CAD build for the part. Positions are in the model's coordinates, mm. A direction names the side the tool comes from. Give positions to 0.01 mm unless a question says otherwise; leave off trailing zeros. Order: outer loops, then holes, each group sorted by start corner. A loop starts at its lowest first (then second) coordinate and runs counter-clockwise, first axis right, second up.
from build123d import *

# Parameters (mm, degrees)
F0_R     = 4.7625
F0_R_2   = 6.35
F1_DEPTH = 12.7


with BuildPart() as f1:
    # F0 (on Front) → F1 (new body)
    with BuildSketch(Plane.XZ):
        with BuildLine():
            ThreePointArc((8.594672, 44.651487), (8.337428, 45.27728), (8.254523, 45.948784))
            ThreePointArc((8.254523, 45.948784), (0, 54.2925), (-8.254523, 45.948784))
            ThreePointArc((-8.254523, 45.948784), (-8.337428, 45.27728), (-8.594672, 44.651487))
            Line((-8.594672, 44.651487), (-42.966658, -14.882539))
            ThreePointArc((-42.966658, -14.882539), (-43.379988, -15.418216), (-43.920076, -15.825765))
            ThreePointArc((-43.920076, -15.825765), (-47.018684, -27.14625), (-35.665553, -30.123019))
            ThreePointArc((-35.665553, -30.123019), (-35.042561, -29.859064), (-34.371986, -29.768948))
            Line((-34.371986, -29.768948), (34.371986, -29.768948))
            ThreePointArc((34.371986, -29.768948), (35.042561, -29.859064), (35.665553, -30.123019))
            ThreePointArc((35.665553, -30.123019), (47.018684, -27.14625), (43.920076, -15.825765))
            ThreePointArc((43.920076, -15.825765), (43.379988, -15.418216), (42.966658, -14.882539))
            Line((42.966658, -14.882539), (8.594672, 44.651487))
        make_face()
        with Locations((-39.869645, -23.01875)):
            Circle(F0_R, mode=Mode.SUBTRACT)
        with Locations((39.869645, -23.01875)):
            Circle(F0_R, mode=Mode.SUBTRACT)
        Circle(F0_R_2, mode=Mode.SUBTRACT)
        with Locations((0, 46.0375)):
            Circle(F0_R, mode=Mode.SUBTRACT)
    extrude(amount=F1_DEPTH)


solid = f1.part
1. Saw through at B-B on z = 0. Give the cut face in (x, y).
2. 3-axis set-ups, long thin cutter, end or side, ignore diameter. For faces 4 (the flat face through (0, -6, -29.769)), 5 (the cylindrical face through (46.93, -6.26, -27.3)): which of +Z, -Z, +X, -X, +Y, -Y reach the whole face in a straight line?
3. Mould opens along Z. For faces 1 (the flat face through (-1, -12.7, -7)), 2 (the cylindrical face through (35.11, -6.26, -22.81)), 3 (the flat face through (26.02, -6.26, 14.47)) say: released by +Z, released by -Z, zero draft, split by the parting line, or undercut.
4. Saw through at A-A on x = 0. State how many separate pieces and enclosed holes the cut face has, plus the area to 3 significant figures.
5. Wall check: line 1 (Z direction, x = -3, y = -2.25); line 2 (X direction, y = -7.25, z = -1.5); line 3 (X direction, y = -4, z = -22). Give the ranges that are in metal, low to high.
6. Pin check, flat tips, straight feed: P1, Ø4, axis at x = -29, y = -4, coming from the +Z side; P2, Ø6.5, axis at x = -11, y = -6, coming from the -Z side; P3, Ø1, axis at y = -4.5, z = -1, coming from the +X side. Stop position of each tip, or through.
7. Saw through at C-C on x = 37. Give the cut face in (y, z).
Reported:
1. outline: (-34.37, -12.7) - (-6.35, -12.7) - (-6.35, 0) - (-34.37, 0) - close; (6.35, -12.7) - (34.37, -12.7) - (34.37, 0) - (6.35, 0) - close
2. face 4: -Z, +Y, -Y
2. face 5: +Y, -Y
3. face 1: zero draft
3. face 2: undercut
3. face 3: released by +Z
4. separate pieces: 3
4. enclosed holes: 0
4. area: 785 mm2
5. line 1: z = -29.77 to -5.6, 5.6 to 42.34, 49.74 to 53.73
5. line 2: x = -35.24 to -6.17, 6.17 to 35.24
5. line 3: x = -48.06 to -44.52, -35.22 to 35.22, 44.52 to 48.06
6. P1: stops at z = 12.77
6. P2: stops at z = -29.77
6. P3: stops at x = 35.24
7. outline: (-12.7, -30.76) - (0, -30.76) - (0, -26.82) - (-12.7, -26.82) - close; (-12.7, -19.22) - (0, -19.22) - (0, -4.55) - (-12.7, -4.55) - close
